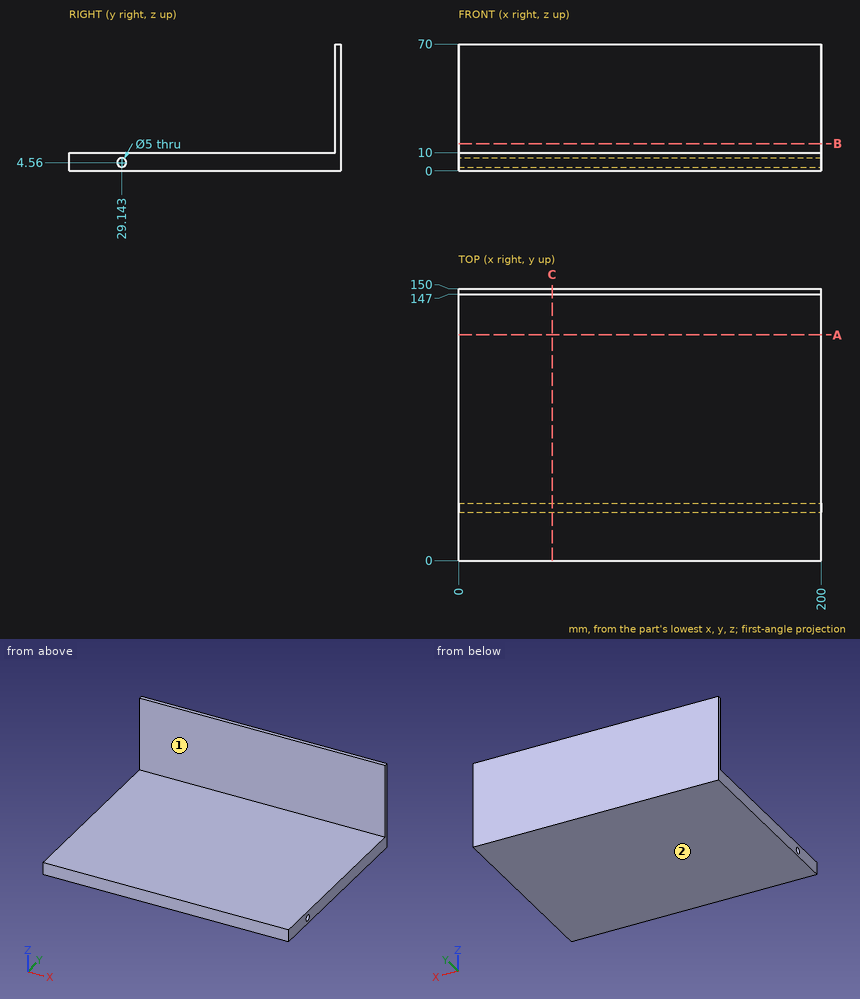
Can you work these out from the drawing? Everything is in mm from the part's minimum corner. A direction names the side the tool comes from. Round coordinates to 2 decimals unless told otherwise and drop trailing zeros. Write each loop counter-clockwise with the first axis right and the second up, starting at its lowest first coordinate (ties: lowest second). Pieces come first, ordered by that corner, then holes.
1. For the marked faces 1 and 2, which set-ups out of +Z, -Z, +X, -X, +Y, -Y let a thin tool reach every point of the face, with its end or its side?
2. Suppose I cut it at C-C (x = 51.5). List the corners of the cut face in (y, z) for me.
3. I need wall thicknesses on L1, parallel to Y at x = 155.5, z = 18; L2, parallel to Z at x = 125, y = 135. Which ranges of each line are inside material? Lowest first, please.
4. Suppose I cut it at B-B (z = 15). List the corners of the cut face in (x, y) for me.
5. Will these pins go through, and if not, where does the flat tip stop? pin 1 Ø3 at (y, z) = (29.14, 4.56) entering from -X; pin 2 Ø5 at (x, y) = (155, 101.5) entering from -Z; pin 3 Ø6 at (x, y) = (22, 107.5) entering from +Z; pin 4 Ø1.5 at (x, z) = (114, 19.5) entering from -Y.
6. Suppose I cut it at A-A (y = 124.5). List the corners of the cut face in (x, z) for me, and give its area (3 significant figures).
Answer sheet:
1. face 1: +Z, +X, -X, -Y
1. face 2: -Z, +X, -X, +Y, -Y
2. outline: (0, 0) - (150, 0) - (150, 70) - (147, 70) - (147, 10) - (0, 10) - close; hole circle Ø5 at (29.14, 4.56)
3. L1: y = 147 to 150
3. L2: z = 0 to 10
4. outline: (0, 147) - (200, 147) - (200, 150) - (0, 150) - close
5. pin 1: passes through
5. pin 2: stops at z = 0
5. pin 3: stops at z = 10
5. pin 4: stops at y = 147
6. outline: (0, 0) - (200, 0) - (200, 10) - (0, 10) - close
6. area: 2,000 mm2
